```python
from build123d import *

# Parameters (mm, degrees)
F1_DEPTH = 952.5
F2_W     = 101.6
F2_H     = 787.4
F2_R     = 14.2875
F3_DEPTH = 63.5
F4_W     = 368.3
F4_H     = 184.15
F4_R     = 20.6375
F4_W_2   = 247.65
F5_DEPTH = 25.4
F8_DEPTH = 12.7


with BuildPart() as f1:
    # F0 (on Right) → F1 (new body, symmetric)
    with BuildSketch(Plane.YZ):
        with BuildLine():
            Line((400.05, 231.775), (-400.05, 231.775))
            ThreePointArc((-400.05, 231.775), (-422.5006403027, 222.4756403027), (-431.8, 200.025))
            Line((-431.8, 200.025), (-431.8, -200.025))
            ThreePointArc((-431.8, -200.025), (-437.3796158184, -213.4953841816), (-450.85, -219.075))
            Line((-450.85, -219.075), (-558.8, -219.075))
            Line((-558.8, -219.075), (-558.8, -231.775))
            Line((-558.8, -231.775), (-450.85, -231.775))
            ThreePointArc((-450.85, -231.775), (-428.3993596973, -222.4756403027), (-419.1, -200.025))
            Line((-419.1, -200.025), (-419.1, 200.025))
            ThreePointArc((-419.1, 200.025), (-413.5203841816, 213.4953841816), (-400.05, 219.075))
            Line((-400.05, 219.075), (400.05, 219.075))
            ThreePointArc((400.05, 219.075), (413.5203841816, 213.4953841816), (419.1, 200.025))
            Line((419.1, 200.025), (419.1, -200.025))
            ThreePointArc((419.1, -200.025), (428.3993596973, -222.4756403027), (450.85, -231.775))
            Line((450.85, -231.775), (558.8, -231.775))
            Line((558.8, -231.775), (558.8, -219.075))
            Line((558.8, -219.075), (450.85, -219.075))
            ThreePointArc((450.85, -219.075), (437.3796158184, -213.4953841816), (431.8, -200.025))
            Line((431.8, -200.025), (431.8, 200.025))
            ThreePointArc((431.8, 200.025), (422.5006403027, 222.4756403027), (400.05, 231.775))
        make_face()
    extrude(amount=F1_DEPTH, both=True)

    # F2 (on face) → F3 (join)
    with BuildSketch(Plane.XY.offset(231.775)):
        with Locations((889, -76.2)):
            Rectangle(F2_W, F2_H)
        with Locations((885.952, -234.95)):
            Circle(F2_R, mode=Mode.SUBTRACT)
        with Locations((885.952, 234.95)):
            Circle(F2_R, mode=Mode.SUBTRACT)
        with Locations((552.704, -76.2)):
            Rectangle(F2_W, F2_H)
        with Locations((555.752, -234.95)):
            Circle(F2_R, mode=Mode.SUBTRACT)
        with Locations((555.752, 234.95)):
            Circle(F2_R, mode=Mode.SUBTRACT)
    extrude(amount=F3_DEPTH)

    # F4 (on face) → F5 (join)
    with BuildSketch(Plane.XY.offset(231.775)):
        with Locations((282.702, -301.625)):
            Rectangle(F4_W, F4_H)
        with Locations((333.502, -317.5)):
            Circle(F4_R, mode=Mode.SUBTRACT)
        with Locations((-488.823, -301.625)):
            Rectangle(F4_W_2, F4_H)
        with Locations((-479.298, -317.5)):
            Circle(F4_R, mode=Mode.SUBTRACT)
        with Locations((-488.823, 301.625)):
            Rectangle(F4_W_2, F4_H)
        with Locations((-479.298, 317.5)):
            Circle(F4_R, mode=Mode.SUBTRACT)
        with Locations((282.702, 301.625)):
            Rectangle(F4_W, F4_H)
        with Locations((333.502, 317.5)):
            Circle(F4_R, mode=Mode.SUBTRACT)
    extrude(amount=F5_DEPTH)

    # F7 (on offset) → F8 (join)
    with BuildSketch(Plane.YZ.offset(800.1)):
        Polygon((400.05, 219.075), (-400.05, 219.075), (-419.1, 200.025), (-419.1, -231.775), (419.1, -231.775), (419.1, 200.025), align=None)
    extrude(amount=-F8_DEPTH)


solid = f1.part
```
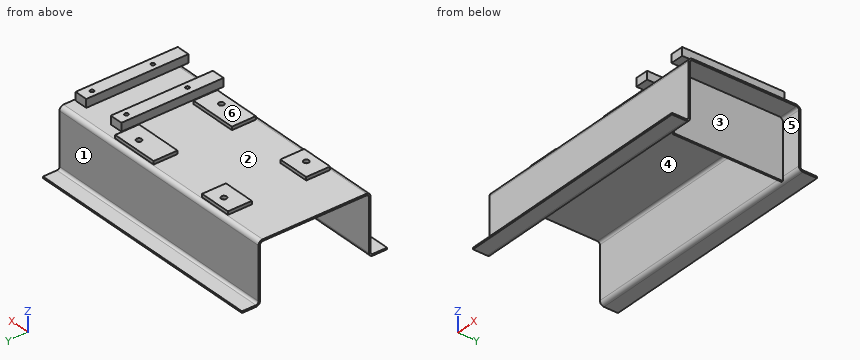
Could you check a few things on this model? Use its own coordinates, in mm. Face numbers are marked on the shaded views. A direction names the side the tool comes from. Give positions to 0.01 mm unless a question says otherwise; leave off trailing zeros. Order: outer loops, then holes, each group sorted by start corner. A loop starts at its lowest first (then second) coordinate and runs counter-clockwise, first axis right, second up.
Q1. We'd pull the mould along X, two halves only. Please class the marked faces 1, 2 and 3: +X half, -X half, draft (parallel to the pull), parting line (faces both ways), or undercut.
Q2. Suppose I cut it at B-B, the plane z = 151.5. Write out the boundary of the cut face in (x, y).
Q3. For the marked faces 4, 5 and 6, which set-ups out of +Z, -Z, +X, -X, +Y, -Y let a thin tool reach every point of the face, with its end or its side?
Q4. Suppose I cut it at C-C, the plane y = -156. Write out the boundary of the cut face in (x, z) (3 decimals), and give its area (3 significant figures).
Q5. I'm going to push flat-ended pins straight in: P1, Ø7.5, axis at x = -480, z = 247, coming from the -Y side; P2, Ø4, axis at y = -219.5, z = -22, coming from the +X side; P3, Ø5, axis at x = 280.5, y = -437.5, coming from the +Z side. Where does each tip first touch, or does it pass through?
Q6. If I drill on line 1 along X through (y, z) = (-276, 234.5); line 2 along X through (y, z) = (234, 254); line 3 along Y through (x, z) = (293.5, 81.5), over which ranges is the centre line in solid material (lowest first)?
Solution:
1. face 1: draft
1. face 2: undercut
1. face 3: +X half
2. outline: (-952.5, -431.8) - (952.5, -431.8) - (952.5, -419.1) - (800.1, -419.1) - (800.1, 419.1) - (952.5, 419.1) - (952.5, 431.8) - (-952.5, 431.8) - (-952.5, 419.1) - (787.4, 419.1) - (787.4, -419.1) - (-952.5, -419.1) - close
3. face 4: -Z, -X
3. face 5: -Z, +X
3. face 6: +Z, -X, +Y, -Y
4. outline: (-952.5, 219.075) - (787.4, 219.075) - (787.4, -231.775) - (800.1, -231.775) - (800.1, 219.075) - (952.5, 219.075) - (952.5, 231.775) - (939.8, 231.775) - (939.8, 295.275) - (838.2, 295.275) - (838.2, 231.775) - (603.504, 231.775) - (603.504, 295.275) - (501.904, 295.275) - (501.904, 231.775) - (-952.5, 231.775) - close
4. area: 42,800 mm2
5. P1: stops at y = -393.7
5. P2: stops at x = 800.1
5. P3: stops at z = -210.59
6. line 1: x = -612.65 to -365, 98.55 to 466.85, 501.9 to 603.5, 838.2 to 939.8
6. line 2: x = -612.65 to -365, 98.55 to 466.85, 501.9 to 541.5, 570.01 to 603.5, 838.2 to 871.7, 900.21 to 939.8
6. line 3: y = -431.8 to -419.1, 419.1 to 431.8
